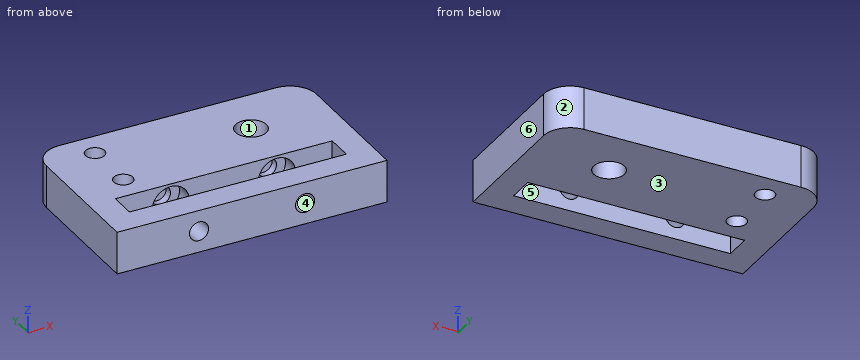
from build123d import *

# Parameters (mm, degrees)
ESQUISSE1_W             = 50.9
ESQUISSE1_H             = 30
ESQUISSE1_R             = 2.9
ESQUISSE1_W_2           = 40.9
ESQUISSE1_H_2           = 5
BOSS_EXTRU_1_DEPTH      = 8
ESQUISSE2_R             = 1.8
ENL_V_MAT_EXTRU_1_DEPTH = 15
CONG_1_R                = 5
ESQUISSE3_R             = 1.8
ENL_V_MAT_EXTRU_2_DEPTH = 10
ESQUISSE4_R             = 3.5
ENL_V_MAT_EXTRU_3_DEPTH = 3.5


with BuildPart() as part:
    # Esquisse1 → Boss.-Extru.1 (new body)
    with BuildSketch(Plane.XY):
        with Locations((25.45, 15)):
            Rectangle(ESQUISSE1_W, ESQUISSE1_H)
        with Locations((35.9, 20)):
            Circle(ESQUISSE1_R, mode=Mode.SUBTRACT)
        with Locations((25.45, 7.5)):
            Rectangle(ESQUISSE1_W_2, ESQUISSE1_H_2, mode=Mode.SUBTRACT)
    extrude(amount=BOSS_EXTRU_1_DEPTH)

    # Esquisse2 → Enlèv. mat.-Extru.1 (cut)
    with BuildSketch(Plane.XZ):
        with Locations(Location((15.45, 4, 0), (0, 0, 270))):
            Circle(ESQUISSE2_R)
        with Locations(Location((35.45, 4, 0), (0, 0, 270))):
            Circle(ESQUISSE2_R)
    extrude(amount=-ENL_V_MAT_EXTRU_1_DEPTH, mode=Mode.SUBTRACT)

    # Congé1
    cong_1_edges = [part.edges().sort_by_distance(p)[0] for p in [
        (0, 30, 4),
        (50.9, 30, 4),
    ]]
    fillet(cong_1_edges, radius=CONG_1_R)

    # Esquisse3 → Enlèv. mat.-Extru.2 (cut)
    with BuildSketch(Plane(origin=(0, 0, 0), x_dir=(-1, 0, 0), z_dir=(0, 0, -1))):
        with Locations((-9.15, 25)):
            Circle(ESQUISSE3_R)
        with Locations((-9.15, 15)):
            Circle(ESQUISSE3_R)
    extrude(amount=-ENL_V_MAT_EXTRU_2_DEPTH, mode=Mode.SUBTRACT)

    # Esquisse4 → Enlèv. mat.-Extru.3 (cut)
    with BuildSketch(Plane.XZ.offset(-10)):
        with Locations((15.45, 4)):
            Circle(ESQUISSE4_R)
        with Locations((35.45, 4)):
            Circle(ESQUISSE4_R)
    extrude(amount=-ENL_V_MAT_EXTRU_3_DEPTH, mode=Mode.SUBTRACT)


solid = part.part
Here's how the part is built. I have some questions about the finished solid (model axes, mm). Face numbers are marked on the shaded views. A direction names the side the tool comes from. Coordinates: 2 decimals unless noted, no trailing zeros. Write each loop counter-clockwise with the first axis right and the second up, starting at its lowest first coordinate (ties: lowest second). Pieces come first, ordered by that corner, then holes.
Item 1: I want a section at B-B on y = 20. Write out the boundary of the cut face in (x, z), and give its area (3 significant figures).
Item 2: I want a section at D-D on z = 4. Count the separate pieces of the cut face and the enclosed holes in it, and give its area (3 significant figures).
Item 3: If we mould it in two halves opening along X, with no side actions, what happens to the marked faces 1, 2 and 3? For each: +X half, -X half, draft (parallel to the pull), parting line (faces both ways), or undercut.
Item 4: Will these pins go through, and if not, where does the flat tip stop? pin 1 (1.1 mm diameter, centred on x = 35.5, z = 4, fed in from -Y); pin 2 (3 mm diameter, centred on x = 9.15, y = 15, fed in from -Z); pin 3 (6 mm diameter, centred on x = 9.15, y = 25, fed in from +Z).
Item 5: I want a section at A-A on x = 15.45. Write out the boundary of the cut face in (y, z), and give its area (3 significant figures).
Item 6: I want a section at C-C on x = 9.15. Write out the boundary of the cut face in (y, z).
Item 7: If I drill on line 1 (Y direction, x = 9.15, z = 4.5); line 2 (Y direction, x = 19, z = 4); line 3 (X direction, y = 12, z = 6.25), over which ranges is the centre line in solid material (lowest first)?
Item 8: On a 3-axis mill with a long thin cutter (end or side, diameter ignored), from which of +Z, -Z, +X, -X, +Y, -Y can I reach the whole of each face in a straight line? I mean the marked faces 4, 5 and 6. Say none if no direction works.
Findings below:
1. outline: (0, 0) - (33, 0) - (33, 8) - (0, 8) - close; (38.8, 0) - (50.9, 0) - (50.9, 8) - (38.8, 8) - close
1. area: 361 mm2
2. separate pieces: 2
2. enclosed holes: 3
2. area: 1,170 mm2
3. face 1: undercut
3. face 2: +X half
3. face 3: draft
4. pin 1: stops at y = 15
4. pin 2: passes through
4. pin 3: stops at z = 8
5. outline: (0, 0) - (5, 0) - (5, 2.2) - (0, 2.2) - close; (0, 5.8) - (5, 5.8) - (5, 8) - (0, 8) - close; (10, 0) - (30, 0) - (30, 8) - (10, 8) - (10, 7.5) - (13.5, 7.5) - (13.5, 5.8) - (15, 5.8) - (15, 2.2) - (13.5, 2.2) - (13.5, 0.5) - (10, 0.5) - close
5. area: 152 mm2
6. outline: (0, 0) - (5, 0) - (5, 8) - (0, 8) - close; (10, 0) - (13.2, 0) - (13.2, 8) - (10, 8) - close; (16.8, 0) - (23.2, 0) - (23.2, 8) - (16.8, 8) - close; (26.8, 0) - (30, 0) - (30, 8) - (26.8, 8) - close
7. line 1: y = 0 to 5, 10 to 13.2, 16.8 to 23.2, 26.8 to 30
7. line 2: y = 0 to 5, 10 to 30
7. line 3: x = 0 to 12.77, 18.13 to 32.77, 38.13 to 50.9
8. face 4: -Y
8. face 5: +Z, -Z
8. face 6: +Z, -Z, +X, +Y, -Y
